from build123d import *

# Parameters (mm, degrees)
EXTRUDE_THIN1_DEPTH = 254
FILLET1_R           = 0.889


with BuildPart() as part:
    # Sketch1 → Extrude-Thin1 (new body)
    with BuildSketch(Plane.XY):
        with BuildLine():
            Line((-22.225, 0), (-25.4, 0))
            Line((-25.4, 0), (-25.4, 4.7625))
            ThreePointArc((-25.4, 4.7625), (-24.935032015, 5.885032015), (-23.8125, 6.35))
            Line((-23.8125, 6.35), (-15.875, 6.35))
            ThreePointArc((-15.875, 6.35), (-9.139807909, 9.139807909), (-6.35, 15.875))
            Line((-6.35, 15.875), (-6.35, 23.8125))
            ThreePointArc((-6.35, 23.8125), (-5.885032015, 24.935032015), (-4.7625, 25.4))
            Line((-4.7625, 25.4), (0, 25.4))
            Line((0, 25.4), (0, 22.225))
            Line((0, 22.225), (-0.889, 22.225))
            Line((-0.889, 22.225), (-0.889, 24.511))
            Line((-0.889, 24.511), (-4.7625, 24.511))
            ThreePointArc((-4.7625, 24.511), (-5.256414087, 24.306414087), (-5.461, 23.8125))
            Line((-5.461, 23.8125), (-5.461, 15.875))
            ThreePointArc((-5.461, 15.875), (-8.511189981, 8.511189981), (-15.875, 5.461))
            Line((-15.875, 5.461), (-23.8125, 5.461))
            ThreePointArc((-23.8125, 5.461), (-24.306414087, 5.256414087), (-24.511, 4.7625))
            Line((-24.511, 4.7625), (-24.511, 0.889))
            Line((-24.511, 0.889), (-22.225, 0.889))
            Line((-22.225, 0.889), (-22.225, 0))
        make_face()
    extrude(amount=-EXTRUDE_THIN1_DEPTH)

    # Fillet1
    fillet1_edges = [part.edges().sort_by_distance(p)[0] for p in [
        (-25.4, 0, -127),
        (0, 25.4, -127),
    ]]
    fillet(fillet1_edges, radius=FILLET1_R)


solid = part.part
Work out the finished part from the listing and answer in its coordinate system (mm). A direction names the side the tool comes from. Coordinates: 2 decimals unless noted, no trailing zeros. Loops run counter-clockwise (first coordinate to the right, second up) from the corner with the lowest first, then second, coordinate; pieces in that order, holes last. Notation, with made-up numbers: M -2.5,64.25 L 43.5,64.25 A12 cw 43.5,69.25 Z; hole C 8,58.25 d8. An arc over 180 degrees is marked long. Answer in a Markdown table with one row per item. Add a question column.
1. Find section B-B, the plane y = 20. Write down the section's boundary in (x, z), then the cut area to 3 significant figures.
2. The mould has two halves that part along X. Classify faces 1 (the flat face through (-24.511, 3, -125)), 2 (the flat face through (-20, 6.35, -125)), 3 (the flat face through (-5.461, 20, -125)): pulls with the +X half, pulls with the -X half, needs draft (parallel to the pull), parting line crosses it, or undercut.
3. Consider L1, parallel to X at y = 3.5, z = -86.5; L2, parallel to Y at x = -1.75, z = -185.5; L3, parallel to Y at x = -15.5, z = -227.5. Determine where each line is inside the solid, lowest interval first.
4. A tool of negligible diameter and unlimited length cuts with its end or side. For faces 4 (the flat face through (-6.35, 20, -125)), 5 (the flat face through (-20, 5.461, -125)), 6 (the flat face through (-3, 25.4, -125)), 7 (the flat face through (-3, 24.511, -125)), from which of +Z, -Z, +X, -X, +Y, -Y can it reach the whole face along a straight path? Write none if from no direction.
5. Flat-ended cylindrical pins translate along their axes: P1, Ø0.7, axis at y = 23.5, z = -172.5, coming from the -X side; P2, Ø0.7, axis at x = -23, z = -68.5, coming from the +Y side; P3, Ø1.2, axis at x = -2.5, z = -92.5, coming from the -Y side. Find the tip coordinate at first contact, or state that the pin passes through.
Reported:
| question | item | result |
|---|---|---|
| 1 | outline | M -6.35,-254 L -5.46,-254 L -5.46,0 L -6.35,0 Z |
| 1 | area | 226 mm^2 |
| 2 | face 1 | pulls with the +X half |
| 2 | face 2 | needs draft |
| 2 | face 3 | undercut |
| 3 | L1 | x = -25.4 to -24.51 |
| 3 | L2 | y = 24.51 to 25.4 |
| 3 | L3 | y = 5.47 to 6.36 |
| 4 | face 4 | +Z, -Z, -X, +Y |
| 4 | face 5 | +Z, -Z, +X |
| 4 | face 6 | +Z, -Z, +X, -X, +Y |
| 4 | face 7 | +Z, -Z, -Y |
| 5 | P1 | stops at x = -6.35 |
| 5 | P2 | stops at y = 6.35 |
| 5 | P3 | stops at y = 24.51 |
